from build123d import *

# Parameters (mm, degrees)
F1_DEPTH = 63.5
F3_DEPTH = 25.4
F5_DEPTH = 7.9375
F7_R     = 6.35


with BuildPart() as f1:
    # F0 (on Front) → F1 (new body, symmetric)
    with BuildSketch(Plane.XZ):
        Polygon((22.225, 14.467527), (-41.275, 14.467527), (-41.275, -14.467527), (41.275, -14.467527), (41.275, 14.467527), align=None)
    extrude(amount=F1_DEPTH, both=True)

    # F0 (on Front) → F3 (join, symmetric)
    with BuildSketch(Plane.XZ):
        with BuildLine():
            Line((22.225, 22.057673), (22.225, 14.467527))
            Line((22.225, 14.467527), (41.275, 14.467527))
            Line((41.275, 14.467527), (41.275, 22.057673))
            ThreePointArc((41.275, 22.057673), (45.92468, 33.282993), (57.15, 37.932673))
            Line((57.15, 37.932673), (63.412444, 37.932673))
            Line((63.412444, 37.932673), (63.412444, 56.982673))
            Line((63.412444, 56.982673), (57.15, 56.982673))
            ThreePointArc((57.15, 56.982673), (32.454296, 46.753377), (22.225, 22.057673))
        make_face()
        Polygon((89.267325, 56.982673), (63.412444, 56.982673), (63.412444, 37.932673), (66.957286, 37.932673), (89.267325, 37.932673), align=None)
    extrude(amount=F3_DEPTH, both=True)

    # F0 (on Front) → F5 (join, symmetric)
    with BuildSketch(Plane.XZ):
        with BuildLine():
            add(Edge.make_bspline(
                [(-41.275, 14.467527), (-18.026909, 45.974523), (22.888102, 66.229478), (57.15, 56.982673)],
                knots=[0, 0, 0, 0, 107.214823, 107.214823, 107.214823, 107.214823], degree=3))
            Line((-41.275, 14.467527), (22.225, 14.467527))
            Line((22.225, 14.467527), (22.225, 22.057673))
            ThreePointArc((22.225, 22.057673), (32.454296, 46.753377), (57.15, 56.982673))
        make_face()
    extrude(amount=F5_DEPTH, both=True)

    # F0 (on Front) → F6 (revolve)
    with BuildSketch(Plane.XZ):
        Polygon((89.267325, 61.732473), (89.267325, 56.982673), (89.267325, 37.932673), (89.267325, 33.157473), (114.212444, 33.157473), (114.212444, 61.732473), align=None)
    revolve(axis=Axis((89.267325, 0, 47.444973), (0, 0, 1)))

    # F7
    f7_edges = [f1.edges().sort_by_distance(p)[0] for p in [
        (-41.275, -63.5, 0),
        (41.275, -63.5, 0),
        (41.275, 63.5, 0),
        (-41.275, 63.5, 0),
    ]]
    fillet(f7_edges, radius=F7_R)


solid = f1.part
Input: part model. Units: mm. Frame: model coordinates. A direction names the side the tool comes from. Coordinates: 2 decimals unless noted, no trailing zeros. Order: outer loops, then holes, each group sorted by start corner. A loop starts at its lowest first (then second) coordinate and runs counter-clockwise, first axis right, second up. Notation, with made-up numbers: M -20,12.25 L -6,12.25 A25 cw -6,32.25 Z; hole C -22.75,48.5 d10. An arc over 180 degrees is marked long. Write item = value, one per line. Start each with the question number.
(1) First-contact query: P1, Ø5, axis at y = -5, z = 31, coming from the +X side; P2, Ø4, axis at y = 30.5, z = 0, coming from the +X side (3 decimals); P3, Ø2, axis at x = 81.5, y = -14.5, coming from the -Z side. Flat tips, straight axial feed; report the tip coordinate or a pass-through.
(2) Reachability of faces 4 (the flat face through (55, -25.4, 41)), 5 (the cylindrical face through (32.727, 16.547, 47.023)), 6 (the flat face through (41.275, -1, 4)) from +Z, -Z, +X, -X, +Y, -Y: full face, straight path, thin tool, end or side. Return the list, or none.
(3) Section B-B on x = 62. Output: boundary loops of the cut face in (y, z), and give its area (3 significant figures).
(4) Section A-A on z = 3.5. Output: boundary loops of the cut face in (x, y) (3 decimals), and give its area (3 significant figures).
(5) Section D-D on y = 23. Output: boundary loops of the cut face in (x, z) (3 decimals).
(6) Line query: line 1 along Z through (x, y) = (21, -35); line 2 along Z through (x, y) = (59, 9); line 3 along Y through (x, z) = (61, 46.5). Output: solid intervals per line, ascending. Write a range as [from, to].
(7) Section C-C on y = -21.5. Output: boundary loops of the cut face in (x, z) (3 decimals), and give its area (3 significant figures).
(8) Pull-direction query (X, two-part tool) for faces 1 (the flat face through (55, 25.4, 41)), 2 (the cylindrical face through (39.464, 61.59, 0.203)), 3 (the flat face through (63, 0, 56.983)); classes: released by +X, released by -X, zero draft, split by the parting line, or undercut.
Result set:
q1.P1 = 113.93
q1.P2 = 41.275
q1.P3 = 33.16
q2.face_4 = +Z, +X, -X, -Y
q2.face_5 = +Z, -X, +Y
q2.face_6 = -Z, +X, +Y, -Y
q3.outline = M -25.4,37.93 L 25.4,37.93 L 25.4,56.98 L -25.4,56.98 Z
q3.area = 968 mm²
q4.outline = M -41.275,-57.15 A6.35 ccw -34.925,-63.5 L 34.925,-63.5 A6.35 ccw 41.275,-57.15 L 41.275,57.15 A6.35 ccw 34.925,63.5 L -34.925,63.5 A6.35 ccw -41.275,57.15 Z
q4.area = 10,400 mm²
q5.outline = M -41.275,-14.468 L 41.275,-14.468 L 41.275,22.058 A15.875 cw 57.15,37.933 L 79.61,37.933 L 79.61,33.157 L 98.924,33.157 L 98.924,61.732 L 79.61,61.732 L 79.61,56.983 L 57.15,56.983 A34.925 ccw 22.225,22.058 L 22.225,14.468 L -41.275,14.468 Z
q6.line_1 = [-14.47, 14.47]
q6.line_2 = [37.93, 56.98]
q6.line_3 = [-25.4, 25.4]
q7.outline = M -41.275,-14.468 L 41.275,-14.468 L 41.275,22.058 A15.875 cw 57.15,37.933 L 76.618,37.933 L 76.618,33.157 L 101.917,33.157 L 101.917,61.732 L 76.618,61.732 L 76.618,56.983 L 57.15,56.983 A34.925 ccw 22.225,22.058 L 22.225,14.468 L -41.275,14.468 Z
q7.area = 4,390 mm²
q8.face_1 = zero draft
q8.face_2 = released by +X
q8.face_3 = undercut
